Verification items for the finished model (mm, model axes). Face numbers are marked on the shaded views. A direction names the side the tool comes from. Give positions to 0.01 mm unless a question says otherwise; leave off trailing zeros. Write each loop counter-clockwise with the first axis right and the second up, starting at its lowest first coordinate (ties: lowest second). Pieces come first, ordered by that corner, then holes. Notation, with made-up numbers: (51, 40.5) -> (105, 40.5) arc R23 cw to (105, 57.5) -> close; hole circle Ø3 at (-24, 79.25). An arc over 180 degrees is marked (long way). Use CSV: the item, a comma, the result in double quotes. Start each with the question number.
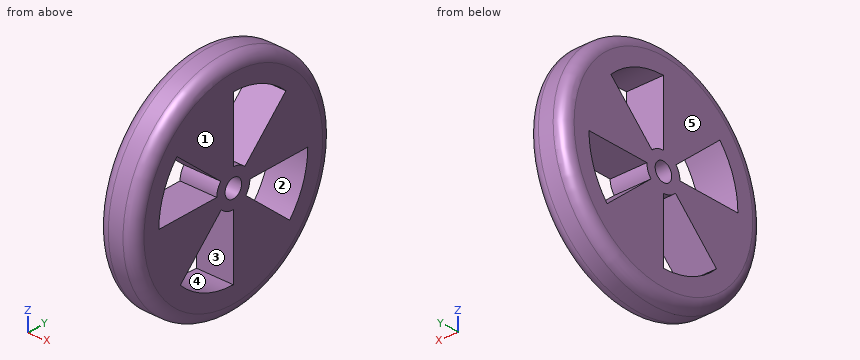
```python
from build123d import *

# Parameters (mm, degrees)
F0_R     = 76.2
F1_DEPTH = 25.4
F2_R     = 6.35
F3_DEPTH = 25.4
F5_DEPTH = 25.4
F6_R     = 7.62


with BuildPart() as f1:
    # F0 (on Right) → F1 (new body)
    with BuildSketch(Plane.YZ):
        Circle(F0_R)
    extrude(amount=F1_DEPTH)

    # F2 (on face) → F3 (cut)
    with BuildSketch(Plane.YZ.offset(25.4)):
        Circle(F2_R)
    extrude(amount=-F3_DEPTH, mode=Mode.SUBTRACT)

    # F4 (on face) → F5 (cut)
    with BuildSketch(Plane.YZ.offset(25.4)):
        with BuildLine():
            ThreePointArc((-40.737736199, -40.0819080058), (-22.0844001217, -52.7105470591), (0, -57.15))
            Line((0, -57.15), (0, -12.7))
            ThreePointArc((0, -12.7), (-5.0078416892, -11.6709691807), (-9.2041521286, -8.7506333253))
            Line((-9.2041521286, -8.7506333253), (-40.737736199, -40.0819080058))
        make_face()
        with BuildLine():
            ThreePointArc((43.2249520119, -37.3861742301), (53.5557116818, -19.947637611), (57.15, 0))
            Line((57.15, 0), (12.7, 0))
            ThreePointArc((12.7, 0), (11.89277789, -4.4555397045), (9.5737269199, -8.3446841081))
            Line((9.5737269199, -8.3446841081), (43.2249520119, -37.3861742301))
        make_face()
        with BuildLine():
            Line((8.8096923922, 9.1476401304), (40.3432764626, 40.4789148108))
            ThreePointArc((40.3432764626, 40.4789148108), (21.8260454338, 52.8180484373), (0, 57.15))
            Line((0, 57.15), (0, 12.7))
            ThreePointArc((0, 12.7), (4.749472094, 11.7784767618), (8.8096923922, 9.1476401304))
        make_face()
        with BuildLine():
            Line((-9.6552608984, 8.2502082994), (-43.3064859904, 37.2916984215))
            ThreePointArc((-43.3064859904, 37.2916984215), (-53.57745876, 19.889153145), (-57.15, 0))
            Line((-57.15, 0), (-12.7, 0))
            ThreePointArc((-12.7, 0), (-11.9145250306, 4.3970550708), (-9.6552608984, 8.2502082994))
        make_face()
    extrude(amount=-F5_DEPTH, mode=Mode.SUBTRACT)

    # F6
    f6_edges = [f1.edges().sort_by_distance(p)[0] for p in [
        (25.4, -76.2, 0),
        (0, -76.2, 0),
    ]]
    fillet(f6_edges, radius=F6_R)


solid = f1.part
```
(1) Draft check along Z on the marked faces 3, 4 and 5. Enter one of: released by +Z, released by -Z, zero draft, split by the parting line, or undercut.
(2) Set-up check for the marked faces 1 and 2: record each of +Z, -Z, +X, -X, +Y, -Y from which the full face is reachable in a straight line by a thin tool's end or side.
(3) Section check B-B on z = 16. Give the number of separate pieces and of enclosed holes in the cut face, then the cut area to 3 significant figures.
(4) Thickness scan on line 1 (Y direction, x = 6.25, z = -15); line 2 (Z direction, x = 20.5, y = 20.5); line 3 (Y direction, x = 1.75, z = 14). Record the ranges inside material, lowest first. Write a range as from..to.
(5) Section check D-D on x = 22. Record the cut outline in (y, z).
(6) Go/stop test with flat-tipped pins: pin 1 (1.5 mm diameter, centred on y = 41, z = 61, fed in from -X); pin 2 (1.5 mm diameter, centred on x = 21.5, z = 55.5, fed in from +Y); pin 3 (10 mm diameter, centred on y = 9, z = 32, fed in from +X); pin 4 (12.5 mm diameter, centred on x = 17.5, y = -24, fed in from +Z). Record where each tip stops, or that it passes through.
(7) Section check A-A on x = 4.75. Record the cut outline in (y, z), then the cut area to 3 significant figures.
Data:
1,face 3,"undercut"
1,face 4,"undercut"
1,face 5,"zero draft"
2,face 1,"+Z, -Z, +X, +Y, -Y"
2,face 2,"+X, -X"
3,separate pieces,"3"
3,enclosed holes,"0"
3,area,"2,410 mm2"
4,line 1,"y = -74.58..-15.49, 0..17.29, 55.15..74.58"
4,line 2,"z = -72.87..-17.77, 0..20.76, 53.35..72.87"
4,line 3,"y = -72.09..-55.41, -16.32..0, 13.69..72.09"
5,outline,"circle Ø149.85 at (0, 0); hole (-57.15, 0) -> (-12.7, 0) arc R12.7 cw to (-9.66, 8.25) -> (-43.31, 37.29) arc R57.15 ccw to start; hole (-40.74, -40.08) arc R57.15 ccw to (0, -57.15) -> (0, -12.7) arc R12.7 cw to (-9.2, -8.75) -> close; hole circle Ø12.7 at (0, 0); hole (0, 12.7) arc R12.7 cw to (8.81, 9.15) -> (40.34, 40.48) arc R57.15 ccw to (0, 57.15) -> close; hole (9.57, -8.34) -> (43.22, -37.39) arc R57.15 ccw to (57.15, 0) -> (12.7, 0) arc R12.7 cw to start"
6,pin 1,"stops at x = 1.24"
6,pin 2,"stops at y = 51.78"
6,pin 3,"passes through"
6,pin 4,"stops at z = 74.1"
7,outline,"circle Ø151.28 at (0, 0); hole (-57.15, 0) -> (-12.7, 0) arc R12.7 cw to (-9.66, 8.25) -> (-43.31, 37.29) arc R57.15 ccw to start; hole (-40.74, -40.08) arc R57.15 ccw to (0, -57.15) -> (0, -12.7) arc R12.7 cw to (-9.2, -8.75) -> close; hole circle Ø12.7 at (0, 0); hole (0, 12.7) arc R12.7 cw to (8.81, 9.15) -> (40.34, 40.48) arc R57.15 ccw to (0, 57.15) -> close; hole (9.57, -8.34) -> (43.22, -37.39) arc R57.15 ccw to (57.15, 0) -> (12.7, 0) arc R12.7 cw to start"
7,area,"13,200 mm2"
